```python
from build123d import *

# Parameters (mm, degrees)
F0_R     = 39.0906
F0_R_2   = 36.5125
F3_R     = 36.5125
F4_DEPTH = 47.498
F5_R     = 39.0906
F5_R_2   = 36.5125
F6_DEPTH = 76.2
F7_R     = 36.5125
F8_DEPTH = 156.718


with BuildPart() as f2:
    # F2: sweep along a path in F1
    with BuildLine(Plane.YZ) as f2_path:
        Line((0, 0), (152.4, 0))
    # F0 (on Front) → F2 (sweep)
    with BuildSketch(Plane.XZ):
        Circle(F0_R)
        Circle(F0_R_2, mode=Mode.SUBTRACT)
    sweep(path=f2_path.line)

    # F3 (on Right) → F4 (cut)
    with BuildSketch(Plane.YZ):
        with Locations((76.2, 0)):
            Circle(F3_R)
    extrude(amount=-F4_DEPTH, mode=Mode.SUBTRACT)

    # F5 (on Right) → F6 (join)
    with BuildSketch(Plane.YZ):
        with Locations((76.2, 0)):
            Circle(F5_R)
        with Locations((76.2, 0)):
            Circle(F5_R_2, mode=Mode.SUBTRACT)
    extrude(amount=-F6_DEPTH)

    # F7 (on Front) → F8 (cut)
    with BuildSketch(Plane.XZ):
        Circle(F7_R)
    extrude(amount=-F8_DEPTH, mode=Mode.SUBTRACT)


solid = f2.part
```
Here's how the part is built. I have some questions about the finished solid (model axes, mm). A direction names the side the tool comes from. Give positions to 0.01 mm unless a question says otherwise; leave off trailing zeros. Order: outer loops, then holes, each group sorted by start corner. A loop starts at its lowest first (then second) coordinate and runs counter-clockwise, first axis right, second up. Notation, with made-up numbers: M 11,14 L 66,14 A12 ccw 66,22 Z; hole C -26.5,-27.5 d8. An arc over 180 degrees is marked long. Use a Markdown table: item, result. Add a question column.
1. Suppose I cut it at A-A (z = 0). List the corners of the cut face in (x, y) for me.
2. I need wall thicknesses on probe 1 along Z at (x, y) = (-58.5, 76.2); probe 2 along X at (y, z) = (138.5, -1); probe 3 along Y at (x, z) = (-27.5, -26.5). Which ranges of each line are inside material? Lowest first, please. Write a range as from..to.
3. Suppose I cut it at C-C (y = 76.2). List the corners of the cut face in (x, z) for me (1 decimal).
4. Suppose I cut it at B-B (x = -22). List the corners of the cut face in (y, z) for me (1 decimal).
5. On a 3-axis mill with a long thin cutter (end or side, diameter ignored), from which of +Z, -Z, +X, -X, +Y, -Y can I reach the whole of each face in a straight line? I mean faces 1 (the flat face through (18, 152.4, 32)), 2 (the cylindrical face through (-46, 112.3, -15)). Say none if no direction works.
6. Suppose I cut it at D-D (y = 34). List the corners of the cut face in (x, z) for me (1 decimal).
7. For pin 1 Ø2 at (y, z) = (93.5, 16) entering from -X; pin 2 Ø10 at (y, z) = (90.5, -7) entering from -X; pin 3 Ø6 at (x, y) = (-18, 55.5) entering from -Z, each with a flat end and sliding along its axis, tell me the tip position at first contact or that it passes through.
8. If we mould it in two halves opening along X, with no side actions, what happens to faces 3 (the cylindrical face through (37.3, 77.3, -11.7)), 4 (the flat face through (18, 0, 32)), 5 (the flat face through (-76.2, 44, 18)), 6 (the cylindrical face through (34.826, 77.267, -10.967))? For each: +X half, -X half, draft (parallel to the pull), parting line (faces both ways), or undercut.
Results list:
| question | item | result |
|---|---|---|
| 1 | outline | M -76.2,37.11 L -39.09,37.11 L -39.09,0 L -36.51,0 L -36.51,39.69 L -76.2,39.69 Z; M -76.2,112.71 L -36.51,112.71 L -36.51,152.4 L -39.09,152.4 L -39.09,115.29 L -76.2,115.29 Z; M 36.51,0 L 39.09,0 L 39.09,152.4 L 36.51,152.4 Z |
| 2 | probe 1 | z = -39.09..-36.51, 36.51..39.09 |
| 2 | probe 2 | x = -39.08..-36.5, 36.5..39.08 |
| 2 | probe 3 | y = 0..51.08, 101.32..152.4 |
| 3 | outline | M -76.2,-39.1 L 0,-39.1 A39.1 ccw 0,39.1 L -76.2,39.1 L -76.2,36.5 L 0,36.5 A36.5 cw 0,-36.5 L -76.2,-36.5 Z |
| 4 | outline | M 0,-32.3 L 54.2,-32.3 A39.1 ccw 98.2,-32.3 L 152.4,-32.3 L 152.4,-29.1 L 98.2,-29.1 A36.5 cw 54.2,-29.1 L 0,-29.1 Z; M 0,29.1 L 54.2,29.1 A36.5 cw 98.2,29.1 L 152.4,29.1 L 152.4,32.3 L 98.2,32.3 A39.1 ccw 54.2,32.3 L 0,32.3 Z |
| 5 | face 1 | +Z, -Z, +X, -X, +Y |
| 5 | face 2 | -X |
| 6 | outline | C 0,0 d78.2; hole C 0,0 d73 |
| 7 | pin 1 | stops at x = 32.31 |
| 7 | pin 2 | stops at x = 34.48 |
| 7 | pin 3 | stops at z = -36.1 |
| 8 | face 3 | parting line |
| 8 | face 4 | draft |
| 8 | face 5 | -X half |
| 8 | face 6 | undercut |
